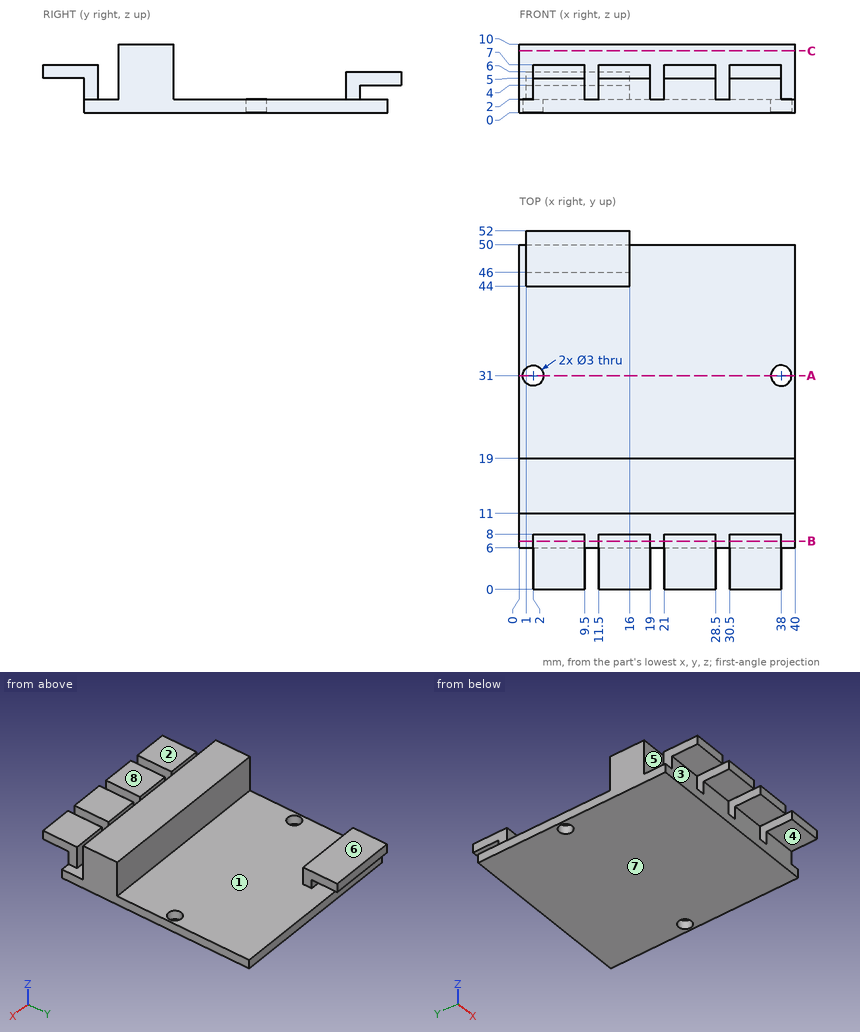
Design review of the part shown in the three views and the two pictorial views. Dimensions are in mm from the part's minimum x, y and z. A direction names the side the tool comes from. Round coordinates to 2 decimals unless told otherwise and drop trailing zeros. Loops run counter-clockwise (first coordinate to the right, second up) from the corner with the lowest first, then second, coordinate; pieces in that order, holes last.
1) Consider section B-B on y = 7. State the section outline as (x, z) points, then the cut area to 3 significant figures.
Values follow:
outline: (0, 0) - (40, 0) - (40, 2) - (38, 2) - (38, 7) - (30.5, 7) - (30.5, 2) - (28.5, 2) - (28.5, 7) - (21, 7) - (21, 2) - (19, 2) - (19, 7) - (11.5, 7) - (11.5, 2) - (9.5, 2) - (9.5, 7) - (2, 7) - (2, 2) - (0, 2) - close
area: 230 mm2
2) Consider section A-A on y = 31. State the section outline as (x, z) points, then the cut area to 3 significant figures.
Values follow:
outline: (0, 0) - (0.5, 0) - (0.5, 2) - (0, 2) - close; (3.5, 0) - (36.5, 0) - (36.5, 2) - (3.5, 2) - close; (39.5, 0) - (40, 0) - (40, 2) - (39.5, 2) - close
area: 68.0 mm2
3) The part is to be moulded in two halves that separate along Y. For the marked faces 1, 2 and 3, say which applies: pulls with the +Y half, pulls with the -Y half, needs draft (parallel to the pull), parting line crosses it, or undercut.
Values follow:
face 1: undercut
face 2: needs draft
face 3: pulls with the -Y half
4) Wall thickness on line 1 along Y through (x, z) = (13, 3); line 2 along Y through (x, z) = (38, 0.85); line 3 along Y through (x, z) = (10, 3.5): over which ranges is each line inside the solid? List them lowest first.
Values follow:
line 1: y = 6 to 8, 11 to 19, 44 to 46
line 2: y = 6 to 29.5, 32.5 to 50
line 3: y = 11 to 19, 44 to 46
5) Consider section C-C on z = 9. State the section outline as (x, y) points, then the cut area to 3 significant figures.
Values follow:
outline: (0, 11) - (40, 11) - (40, 19) - (0, 19) - close
area: 320 mm2
6) Tool access review of the marked faces 4, 5, 6, 7 and 8: name each direction out of +Z, -Z, +X, -X, +Y, -Y from which nothing blocks a thin tool from reaching the whole face with its end or side.
Values follow:
face 4: -Z, +X, -X, -Y
face 5: +Z, +X, -X
face 6: +Z, +X, -X, +Y
face 7: -Z, +X, -X, +Y, -Y
face 8: +Z, +X, -X, -Y
7) Clearance check with flat-ended pins moving along their axes: P1, Ø1.5, axis at x = 30, z = 3, coming from the +Y side; P2, Ø1.2, axis at y = 46, z = 3.5, coming from the -X side; P3, Ø4, axis at y = 5, z = 4, coming from the -X side; P4, Ø3, axis at y = 21, z = 9, coming from the +X side. State where each tip first meets the part, or that it passes through.
Values follow:
P1: stops at y = 19
P2: stops at x = 1
P3: stops at x = 2
P4: passes through
